Work out the finished part from the listing and answer in its coordinate system (mm). A direction names the side the tool comes from. Coordinates: 2 decimals unless noted, no trailing zeros. Order: outer loops, then holes, each group sorted by start corner. A loop starts at its lowest first (then second) coordinate and runs counter-clockwise, first axis right, second up. Notation, with made-up numbers: M -1,74 L 30,74 A23 cw 30,86 Z; hole C 15.5,2.5 d11. An arc over 180 degrees is marked long. Write item = value, one per line. Start each with the question number.
Q1. A tool of negligible diameter and unlimited length cuts with its end or side. For faces 4 (the flat face through (0, -10, 19)), 5 (the flat face through (0, 10, 21.5)), 6 (the flat face through (-11, -4, 2)), from which of +Z, -Z, +X, -X, +Y, -Y can it reach the whole face along a straight path? Write none if from no direction.
Q2. Find section A-A on x = 0. Give the vertices of the cut face in (y, z).
Q3. Find section D-D on x = -3. Give the number of separate pieces and of enclosed holes in the cut face, and give its area (3 significant figures).
Q4. Find section C-C on z = 25. Give the vertices of the cut face in (x, y), and give its area (3 significant figures).
Q5. Each of these flat-tipped pins is pushed along its axis until it touches: P1, Ø4, axis at y = 8, z = 4.5, coming from the +X side; P2, Ø2.5, axis at x = 10, y = 1, coming from the -Z side; P3, Ø12, axis at x = 3, z = 17, coming from the +Y side; P4, Ø3, axis at x = 3, z = 11.5, coming from the -Y side. Where does it stop, or does it pass through?
Q6. Determine the mould class of faces 1 (the cylindrical face through (-8.292, 7.603, 16.05)), 2 (the cylindrical face through (9.465, 4.458, 16.071)), 3 (the cylindrical face through (-5.778, -8.677, 18.316)) for opening direction Y: released by +Y, released by -Y, zero draft, split by the parting line, or undercut.
Q7. Find section B-B on y = 0. Give the vertices of the cut face in (x, z), and give its area (4 significant figures).
Q8. Straight lines are drawn through the part: line 1 along Z through (x, y) = (0, -10.4); line 2 along Z through (x, y) = (-9.5, -3.25); line 3 along X through (y, z) = (0, 23.5). For each, find the intervals that lie inside material, in ascending order.
```python
from build123d import *

# Parameters (mm, degrees)
ESQUISSE1_R             = 11.25
ESQUISSE1_R_2           = 9.5
BASE_EXTRUSION_DEPTH    = 31
CHANFREIN1_SIZE         = 0.5
ESQUISSE2_R             = 12.25
ESQUISSE2_R_2           = 11.25
BOSS_EXTRU_MINCE1_DEPTH = 2
ESQUISSE3_R             = 1.5
ENL_V_MAT_EXTRU_1_DEPTH = 36.512321805
ENL_V_MAT_EXTRU_2_DEPTH = 25
ENL_V_MAT_EXTRU_3_DEPTH = 50


with BuildPart() as part:
    # Esquisse1 → Base-Extrusion (new body)
    with BuildSketch(Plane.XY):
        Circle(ESQUISSE1_R)
        Circle(ESQUISSE1_R_2, mode=Mode.SUBTRACT)
    extrude(amount=BASE_EXTRUSION_DEPTH)

    # Chanfrein1
    chanfrein1_edges = [part.edges().sort_by_distance(p)[0] for p in [
        (-11.25, 0, 31),
    ]]
    chamfer(chanfrein1_edges, length=CHANFREIN1_SIZE)

    # Esquisse2 → Boss.-Extru.-Mince1 (add)
    with BuildSketch(Plane(origin=(0, 0, 0), x_dir=(-1, 0, 0), z_dir=(0, 0, -1))):
        Circle(ESQUISSE2_R)
        Circle(ESQUISSE2_R_2, mode=Mode.SUBTRACT)
    extrude(amount=-BOSS_EXTRU_MINCE1_DEPTH)

    # Esquisse3 → Enlèv. mat.-Extru.1 (cut, through all)
    with BuildSketch(Plane(origin=(0, 0, 0), x_dir=(1, 0, 0), z_dir=(0, 1, 0))):
        with Locations(Location((0, -25, 0), (0, 0, 270))):
            Circle(ESQUISSE3_R)
        with BuildLine():
            Line((-4.1, -14), (4.1, -14))
            ThreePointArc((4.1, -14), (5.797056275, -14.702943725), (6.5, -16.4))
            Line((6.5, -16.4), (6.5, -16.6))
            ThreePointArc((6.5, -16.6), (5.797056275, -18.297056275), (4.1, -19))
            Line((4.1, -19), (-4.1, -19))
            ThreePointArc((-4.1, -19), (-5.797056275, -18.297056275), (-6.5, -16.6))
            Line((-6.5, -16.6), (-6.5, -16.4))
            ThreePointArc((-6.5, -16.4), (-5.797056275, -14.702943725), (-4.1, -14))
        make_face()
    extrude(amount=-ENL_V_MAT_EXTRU_1_DEPTH, mode=Mode.SUBTRACT)

    # Esquisse4 → Enlèv. mat.-Extru.2 (cut, symmetric)
    with BuildSketch(Plane(origin=(0, 0, 0), x_dir=(0, 0, -1), z_dir=(1, 0, 0))):
        with BuildLine():
            Line((-17.6, 5), (-17.4, 5))
            ThreePointArc((-17.4, 5), (-16.056497116, 4.443502884), (-15.5, 3.1))
            Line((-15.5, 3.1), (-15.5, -3.1))
            ThreePointArc((-15.5, -3.1), (-16.056497116, -4.443502884), (-17.4, -5))
            Line((-17.4, -5), (-17.6, -5))
            ThreePointArc((-17.6, -5), (-18.943502884, -4.443502884), (-19.5, -3.1))
            Line((-19.5, -3.1), (-19.5, 3.1))
            ThreePointArc((-19.5, 3.1), (-18.943502884, 4.443502884), (-17.6, 5))
        make_face()
    extrude(amount=ENL_V_MAT_EXTRU_2_DEPTH, both=True, mode=Mode.SUBTRACT)

    # Esquisse5 → Enlèv. mat.-Extru.3 (cut)
    with BuildSketch(Plane(origin=(0, 0, 0), x_dir=(1, 0, 0), z_dir=(0, 1, 0))):
        with BuildLine():
            Line((-2.6, -17.5), (2.6, -17.5))
            ThreePointArc((2.6, -17.5), (3.943502884, -18.056497116), (4.5, -19.4))
            Line((4.5, -19.4), (4.5, -19.6))
            ThreePointArc((4.5, -19.6), (3.943502884, -20.943502884), (2.6, -21.5))
            Line((2.6, -21.5), (-2.6, -21.5))
            ThreePointArc((-2.6, -21.5), (-3.943502884, -20.943502884), (-4.5, -19.6))
            Line((-4.5, -19.6), (-4.5, -19.4))
            ThreePointArc((-4.5, -19.4), (-3.943502884, -18.056497116), (-2.6, -17.5))
        make_face()
    extrude(amount=ENL_V_MAT_EXTRU_3_DEPTH, mode=Mode.SUBTRACT)


solid = part.part
```
Findings below:
q1.face_4 = +Y, -Y
q1.face_5 = +Y
q1.face_6 = +Z
q2.outline = M -12.25,0 L -9.5,0 L -9.5,14 L -11.25,14 L -11.25,2 L -12.25,2 Z; M -11.25,19 L -9.5,19 L -9.5,23.5 L -11.25,23.5 Z; M -11.25,26.5 L -9.5,26.5 L -9.5,31 L -10.75,31 L -11.25,30.5 Z; M 9.5,0 L 12.25,0 L 12.25,2 L 11.25,2 L 11.25,17.5 L 9.5,17.5 Z; M 9.5,21.5 L 11.25,21.5 L 11.25,30.5 L 10.75,31 L 9.5,31 Z
q3.separate_pieces = 4
q3.enclosed_holes = 0
q3.area = 101 mm^2
q4.outline = M -1.5,-11.15 L -1.5,-9.38 A9.5 cw long 1.5,-9.38 L 1.5,-11.15 A11.25 ccw long Z
q4.area = 109 mm^2
q5.P1 = 9.52
q5.P2 = 0
q5.P3 = 11.25
q5.P4 = -11.15
q6.face_1 = split by the parting line
q6.face_2 = undercut
q6.face_3 = zero draft
q7.outline = M -12.25,0 L -9.5,0 L -9.5,15.5 L -11.25,15.5 L -11.25,2 L -12.25,2 Z; M -11.25,19.5 L -9.5,19.5 L -9.5,31 L -10.75,31 L -11.25,30.5 Z; M 9.5,0 L 12.25,0 L 12.25,2 L 11.25,2 L 11.25,15.5 L 9.5,15.5 Z; M 9.5,19.5 L 11.25,19.5 L 11.25,30.5 L 10.75,31 L 9.5,31 Z
q7.area = 98.25 mm^2
q8.line_1 = 0 to 14, 19 to 23.5, 26.5 to 31
q8.line_2 = 0 to 15.51, 19.49 to 31
q8.line_3 = -11.25 to -9.5, 9.5 to 11.25
